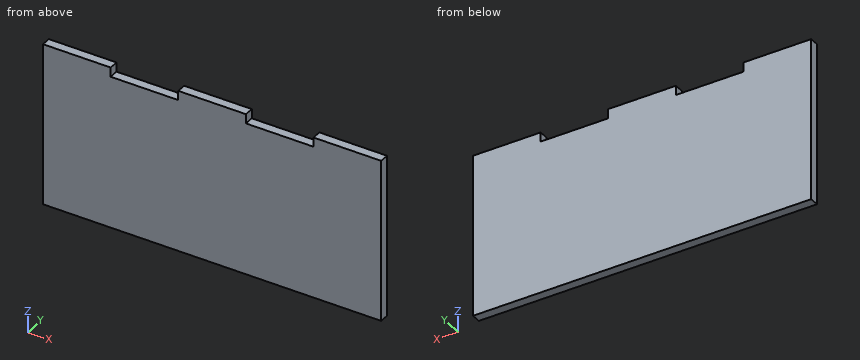
from build123d import *

# Parameters (mm, degrees)
SKETCH1_W           = 354.00488
SKETCH1_H           = 169.3164
BOSS_EXTRUDE1_DEPTH = 9.7536
SKETCH2_W           = 70.800976
SKETCH2_H           = 9.7536
CUT_EXTRUDE1_DEPTH  = 333.802189186


with BuildPart() as part:
    # Sketch1 → Boss-Extrude1 (new body)
    with BuildSketch(Plane(origin=(0, 0, 0), x_dir=(1, 0, 0), z_dir=(0, 1, 0))):
        with Locations((107.281446772, 88.098380587)):
            Rectangle(SKETCH1_W, SKETCH1_H)
    extrude(amount=BOSS_EXTRUDE1_DEPTH)

    # Sketch2 → Cut-Extrude1 (cut, through all)
    with BuildSketch(Plane.XZ):
        with Locations((178.082422772, -8.316980587)):
            Rectangle(SKETCH2_W, SKETCH2_H)
        with Locations((36.480470772, -8.316980587)):
            Rectangle(SKETCH2_W, SKETCH2_H)
    extrude(amount=-CUT_EXTRUDE1_DEPTH, mode=Mode.SUBTRACT)


solid = part.part
Verification items for the finished model (mm, model axes). Round coordinates to 2 decimals unless told otherwise and drop trailing zeros. Loops run counter-clockwise (first coordinate to the right, second up) from the corner with the lowest first, then second, coordinate; pieces in that order, holes last. Notation, with made-up numbers: (70.5, 12.5) - (125.5, 12.5) arc R10 ccw to (125.5, 19.5) - close; hole circle Ø6 at (-11, 59). An arc over 180 degrees is marked (long way). Use one line per item in the form item = value.
1. Section check B-B on x = 54. Record the cut outline in (y, z).
A:
outline = (0, -172.76) - (9.75, -172.76) - (9.75, -13.19) - (0, -13.19) - close
2. Section check A-A on y = 8. Record the cut outline in (x, z), and give its area (3 significant figures).
A:
outline = (-69.72, -172.76) - (284.28, -172.76) - (284.28, -3.44) - (213.48, -3.44) - (213.48, -13.19) - (142.68, -13.19) - (142.68, -3.44) - (71.88, -3.44) - (71.88, -13.19) - (1.08, -13.19) - (1.08, -3.44) - (-69.72, -3.44) - close
area = 58,600 mm²
3. Gauge pin test, flat end, axial feed: pin 1 Ø1.5 at (x, y) = (21, 2) entering from +Z. Record the tip position at first contact, or that the pin passes through.
A:
pin_1 = -13.19
4. Scan line: probe 1 along Z at (x, y) = (209, 8.5). Record every from-to range of solid material in increasing order.
A:
probe_1 = -172.76 to -13.19
